```python
from build123d import *

# Parameters (mm, degrees)
SKETCH_1_W          = 18
SKETCH_1_H          = 126
EXTRUDE_1_DEPTH     = 8
CUT_EXTRUDE_1_DEPTH = 10
FILLET_1_R          = 5
FILLET_2_R          = 2
EXTRUDE_5_DEPTH     = 8
CUT_EXTRUDE_4_DEPTH = 8
FILLET_3_R          = 1
FILLET_4_R          = 1


with BuildPart() as part:
    # 스케치1 → 보스-돌출1 (new body)
    with BuildSketch(Plane(origin=(0, 0, 0), x_dir=(1, 0, 0), z_dir=(0, 1, 0))):
        with Locations((9, 63)):
            Rectangle(SKETCH_1_W, SKETCH_1_H)
    extrude(amount=EXTRUDE_1_DEPTH)

    # 스케치2 → 컷-돌출1 (cut)
    with BuildSketch(Plane(origin=(0, 8, 0), x_dir=(1, 0, 0), z_dir=(0, 1, 0))):
        with BuildLine():
            Line((12.5, 94.25), (18, 94.25))
            ThreePointArc((18, 94.25), (21.25, 91), (18, 87.75))
            Line((18, 87.75), (12.5, 87.75))
            ThreePointArc((12.5, 87.75), (9.25, 91), (12.5, 94.25))
        make_face()
        with BuildLine():
            Line((12.5, 57.25), (18, 57.25))
            ThreePointArc((18, 57.25), (21.25, 54), (18, 50.75))
            Line((18, 50.75), (12.5, 50.75))
            ThreePointArc((12.5, 50.75), (9.25, 54), (12.5, 57.25))
        make_face()
        with BuildLine():
            Line((12.5, 20.25), (18, 20.25))
            ThreePointArc((18, 20.25), (21.25, 17), (18, 13.75))
            Line((18, 13.75), (12.5, 13.75))
            ThreePointArc((12.5, 13.75), (9.25, 17), (12.5, 20.25))
        make_face()
    extrude(amount=-CUT_EXTRUDE_1_DEPTH, mode=Mode.SUBTRACT)

    # 필렛1
    fillet_1_edges = [part.edges().sort_by_distance(p)[0] for p in [
        (18, 4, -126),
    ]]
    fillet(fillet_1_edges, radius=FILLET_1_R)

    # 필렛2
    fillet_2_edges = [part.edges().sort_by_distance(p)[0] for p in [
        (18, 4, -94.25),
        (18, 4, -87.75),
        (18, 4, -57.25),
        (18, 4, -50.75),
        (18, 4, -20.25),
        (18, 4, -13.75),
    ]]
    fillet(fillet_2_edges, radius=FILLET_2_R)

    # 스케치10 → 보스-돌출5 (add)
    with BuildSketch(Plane.XZ):
        with BuildLine():
            Line((9.5, 0), (9.5, 2.820550528))
            ThreePointArc((9.5, 2.820550528), (9.449358869, 3.267764124), (9.3, 3.692330317))
            ThreePointArc((9.3, 3.692330317), (12, 8), (14.7, 3.692330317))
            ThreePointArc((14.7, 3.692330317), (14.550641131, 3.267764124), (14.5, 2.820550528))
            Line((14.5, 2.820550528), (14.5, 0))
            Line((14.5, 0), (9.5, 0))
        make_face()
    extrude(amount=-EXTRUDE_5_DEPTH)

    # 스케치11 → 컷-돌출4 (cut)
    with BuildSketch(Plane.XZ):
        with BuildLine():
            Line((0, -117.5), (2.820550528, -117.5))
            ThreePointArc((2.820550528, -117.5), (3.267764124, -117.449358869), (3.692330317, -117.3))
            ThreePointArc((3.692330317, -117.3), (8, -120), (3.692330317, -122.7))
            ThreePointArc((3.692330317, -122.7), (3.267764124, -122.550641131), (2.820550528, -122.5))
            Line((2.820550528, -122.5), (0, -122.5))
            Line((0, -122.5), (0, -117.5))
        make_face()
    extrude(amount=-CUT_EXTRUDE_4_DEPTH, mode=Mode.SUBTRACT)

    # 필렛3
    fillet_3_edges = [part.edges().sort_by_distance(p)[0] for p in [
        (9.5, 4, 0),
        (14.5, 4, 0),
    ]]
    fillet(fillet_3_edges, radius=FILLET_3_R)

    # 필렛4
    fillet_4_edges = [part.edges().sort_by_distance(p)[0] for p in [
        (0, 4, -122.5),
        (0, 4, -117.5),
    ]]
    fillet(fillet_4_edges, radius=FILLET_4_R)


solid = part.part
```
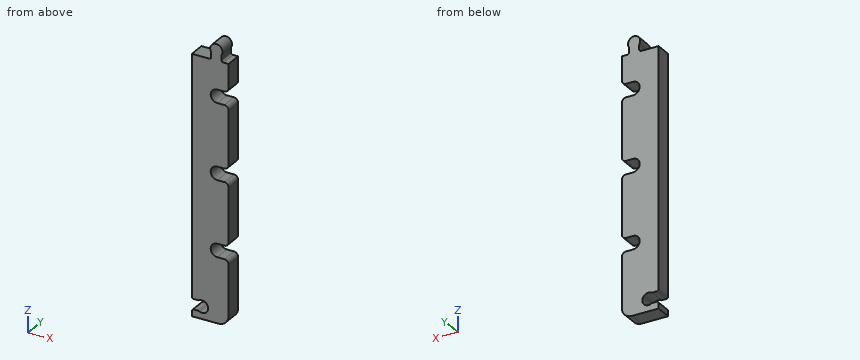
Part model, mm, in its own coordinate system. Coordinates: 2 decimals unless noted, no trailing zeros. Write each loop counter-clockwise with the first axis right and the second up, starting at its lowest first coordinate (ties: lowest second). Pieces come first, ordered by that corner, then holes.
Item 1: Slice it at B-B (z = 5). Write the cut outline in (x, y).
Item 2: Slice it at A-A (z = -91). Write the cut outline in (x, y).
Item 3: Pin check, flat tips, straight feed: pin 1 (1 mm diameter, centred on x = 14, y = 2, fed in from +Z); pin 2 (1.2 mm diameter, centred on x = 17, y = 4, fed in from +Z); pin 3 (1 mm diameter, centred on y = 6, z = -13.5, fed in from +X). Stop position of each tip, or through.
Item 4: Probe line 1 (Z direction, x = 5, y = 3); line 2 (Z direction, x = 13, y = 0.75); line 3 (X direction, y = 1, z = -53.5). List the from-to ranges inside material, lowest first.
Results found:
1. outline: (9, 0) - (15, 0) - (15, 8) - (9, 8) - close
2. outline: (0, 0) - (9.25, 0) - (9.25, 8) - (0, 8) - close
3. pin 1: stops at z = 7.6
3. pin 2: stops at z = 0
3. pin 3: stops at x = 17.56
4. line 1: z = -126 to -123, -117 to 0
4. line 2: z = -126 to -94.25, -87.75 to -57.25, -50.75 to -20.25, -13.75 to 7.83
4. line 3: x = 0 to 9.29
